Here's how the part is built. I have some questions about the finished solid (model axes, mm). Round coordinates to 2 decimals unless told otherwise and drop trailing zeros. Order: outer loops, then holes, each group sorted by start corner. A loop starts at its lowest first (then second) coordinate and runs counter-clockwise, first axis right, second up. Notation, with made-up numbers: M 14,58.25 L 31,58.25 A21 ccw 31,72.25 Z; hole C 4.5,53.25 d2. An arc over 180 degrees is marked long. Use one line per item in the form item = value. Start each with the question number.
```python
from build123d import *

# Parameters (mm, degrees)
SKETCH_1_R      = 1
EXTRUDE_1_DEPTH = 3


with BuildPart() as part:
    # 草图1 → 凸台-拉伸1 (new body)
    with BuildSketch(Plane(origin=(0, 0, 0), x_dir=(1, 0, 0), z_dir=(0, 1, 0))):
        with BuildLine():
            Line((0, 2), (18, 2))
            ThreePointArc((18, 2), (18.083405892, 1.998260107), (18.166666667, 1.993043457))
            Line((18.166666667, 1.993043457), (42, 0))
            Line((42, 0), (18.166666667, -1.993043457))
            ThreePointArc((18.166666667, -1.993043457), (18.083405892, -1.998260107), (18, -2))
            Line((18, -2), (0, -2))
            ThreePointArc((0, -2), (-2, 0), (0, 2))
        make_face()
        Circle(SKETCH_1_R, mode=Mode.SUBTRACT)
        with Locations((18, 0)):
            Circle(SKETCH_1_R, mode=Mode.SUBTRACT)
    extrude(amount=EXTRUDE_1_DEPTH)


solid = part.part
```
1) If we mould it in two halves opening along Z, with no side actions, what happens to faces 1 (the flat face through (30.25, 1.479, 0.983)), 2 (the cylindrical face through (19, 1, 0)), 3 (the cylindrical face through (-2, 1, 0)), 4 (the flat face through (15, 3, 0))? For each: +Z half, -Z half, draft (parallel to the pull), parting line (faces both ways), or undercut.
2) If we section it at C-C on x = 23.5: Write out the boundary of the cut face in (y, z), then the cut area to 3 significant figures.
3) If I drill on line 1 (Z direction, x = 18, y = 2.15); line 2 (Z direction, x = 19.5, y = 2); line 3 (Z direction, x = 32.5, y = 0.55), over which ranges is the centre line in solid material (lowest first)?
4) If we section it at B-B on z = -0.6: Write out the boundary of the cut face in (x, y), then the cut area to 3 significant figures.
5) If we section it at A-A on y = 0.9: Write out the boundary of the cut face in (x, z).
Completed:
q1.face_1 = +Z half
q1.face_2 = undercut
q1.face_3 = parting line
q1.face_4 = draft
q2.outline = M 0,-1.55 L 3,-1.55 L 3,1.55 L 0,1.55 Z
q2.area = 9.28 mm²
q3.line_1 = -2 to -1, 1 to 2
q3.line_2 = -1.88 to 1.88
q3.line_3 = -0.79 to 0.79
q4.outline = M -1.91,0 L -0.8,0 L -0.8,3 L -1.91,3 Z; M 0.8,0 L 17.2,0 L 17.2,3 L 0.8,3 Z; M 18.8,0 L 34.83,0 L 34.83,3 L 18.8,3 Z
q4.area = 101 mm²
q5.outline = M 0,-2 L 18,-2 A2 ccw 18.17,-1.99 L 42,0 L 18.17,1.99 A2 ccw 18,2 L 0,2 A2 ccw Z; hole C 0,0 d2; hole C 18,0 d2
